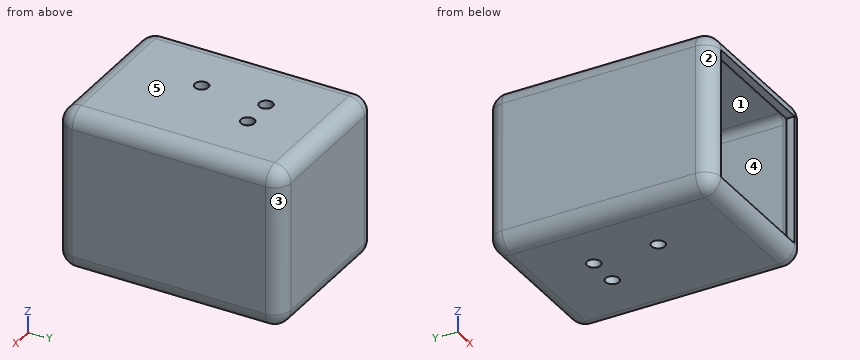
from build123d import *

# Parameters (mm, degrees)
F1_DEPTH = 35
F2_R     = 5
F3_T     = -2.5
F5_D     = 4.2


# Not quite as in the source:
# - a shell that OpenCascade refuses in one call is made with other operations: the cavity is built on its own and cut out


with BuildPart() as f1:
    # F0 (on Front) → F1 (new body, symmetric)
    with BuildSketch(Plane.XZ):
        with BuildLine():
            Line((20, 25), (-20, 25))
            ThreePointArc((-20, 25), (-23.5355339059, 23.5355339059), (-25, 20))
            Line((-25, 20), (-25, -20))
            ThreePointArc((-25, -20), (-23.5355339059, -23.5355339059), (-20, -25))
            Line((-20, -25), (20, -25))
            ThreePointArc((20, -25), (23.5355339059, -23.5355339059), (25, -20))
            Line((25, -20), (25, 20))
            ThreePointArc((25, 20), (23.5355339059, 23.5355339059), (20, 25))
        make_face()
    extrude(amount=F1_DEPTH, both=True)

    # F2
    f2_edges = [f1.edges().sort_by_distance(p)[0] for p in [
        (0, 35, 25),
        (-23.535534, 35, 23.535534),
        (-25, 35, 0),
        (-23.535534, 35, -23.535534),
        (0, 35, -25),
        (23.535534, 35, -23.535534),
        (25, 35, 0),
        (23.535534, 35, 23.535534),
        (0, -35, 25),
        (-23.535534, -35, 23.535534),
        (-25, -35, 0),
        (-23.535534, -35, -23.535534),
        (0, -35, -25),
        (23.535534, -35, -23.535534),
        (25, -35, 0),
        (23.535534, -35, 23.535534),
    ]]
    fillet(f2_edges, radius=F2_R)

    # F3: a shell. OpenCascade refuses it in one call, so the cavity is built on its own and cut out:
    # the body offset inwards by the wall thickness, plus a prism from it out through each open face.
    f3_core = offset(f1.part, amount=F3_T, mode=Mode.PRIVATE)
    f3_exits = [f3_core.faces().sort_by_distance(p)[0] for p in [
        (0, -32.5, 0),
    ]]
    add(f3_core, mode=Mode.SUBTRACT)
    extrude(f3_exits, amount=-F3_T, mode=Mode.SUBTRACT)

    # F5 (through all)
    with Locations(Plane(origin=(0, 0, -25), x_dir=(1, 0, 0), z_dir=(0, 0, -1))):
        with Locations((5, -13), (-5, 7), (-5, -13)):
            Hole(F5_D / 2)


solid = f1.part
For this review, take the finished solid that the model builds, in its own axes (mm). Face numbers are marked on the shaded views. A direction names the side the tool comes from. Round coordinates to 2 decimals unless told otherwise and drop trailing zeros. Write each loop counter-clockwise with the first axis right and the second up, starting at its lowest first coordinate (ties: lowest second). Pieces come first, ordered by that corner, then holes. Notation, with made-up numbers: (-33.75, 24) -> (-18.75, 24) arc R19 ccw to (-18.75, 47) -> close; hole circle Ø11 at (87, 49). An arc over 180 degrees is marked (long way). Put each result on its own line as item: value.
Q1. Clearance check with flat-ended pins moving along their axes: pin 1 Ø2.5 at (x, y) = (-5, -7) entering from +Z; pin 2 Ø0.8 at (x, y) = (-7.5, -33.5) entering from -Z; pin 3 Ø3 at (y, z) = (-34.5, 6) entering from -X; pin 4 Ø3 at (x, y) = (-3, -34) entering from +Z. State where each tip first meets the part, or that it passes through.
Determined:
pin 1: passes through
pin 2: stops at z = -23.92
pin 3: stops at x = -24
pin 4: stops at z = 24.33
Q2. Consider section B-B on x = 5. State the section outline as (y, z) points.
Determined:
outline: (-35, -20) arc R5 ccw to (-30, -25) -> (10.9, -25) -> (10.9, -22.5) -> (-30, -22.5) arc R2.5 cw to (-32.5, -20) -> close; (-35, 20) -> (-32.5, 20) arc R2.5 cw to (-30, 22.5) -> (10.9, 22.5) -> (10.9, 25) -> (-30, 25) arc R5 ccw to start; (15.1, -25) -> (30, -25) arc R5 ccw to (35, -20) -> (35, 20) arc R5 ccw to (30, 25) -> (15.1, 25) -> (15.1, 22.5) -> (30, 22.5) arc R2.5 cw to (32.5, 20) -> (32.5, -20) arc R2.5 cw to (30, -22.5) -> (15.1, -22.5) -> close
Q3. The part is to be moulded in two halves that separate along Z. For the marked faces 3, 4 and 5, say which applies: released by +Z, released by -Z, zero draft, split by the parting line, or undercut.
Determined:
face 3: zero draft
face 4: undercut
face 5: released by +Z
Q4. To check wall thickness, follow L1, parallel to Z at x = 17, y = 10; L2, parallel to X at y = 13, z = -23.95; L3, parallel to Y at x = -5, z = 24. State the ranges of each line that lie inside material, in increasing order. Write a range as [from, to].
Determined:
L1: z = [-25, -22.5], [22.5, 25]
L2: x = [-23.07, -7.1], [-2.9, 2.9], [7.1, 23.07]
L3: y = [-33, -9.1], [-4.9, 10.9], [15.1, 33]
Q5. Consider section A-A on y = -7. State the section outline as (x, z) points, and give its area (3 significant figures).
Determined:
outline: (-25, -20) arc R5 ccw to (-20, -25) -> (-7.1, -25) -> (-7.1, -22.5) -> (-20, -22.5) arc R2.5 cw to (-22.5, -20) -> (-22.5, 20) arc R2.5 cw to (-20, 22.5) -> (-7.1, 22.5) -> (-7.1, 25) -> (-20, 25) arc R5 ccw to (-25, 20) -> close; (-2.9, -25) -> (20, -25) arc R5 ccw to (25, -20) -> (25, 20) arc R5 ccw to (20, 25) -> (-2.9, 25) -> (-2.9, 22.5) -> (20, 22.5) arc R2.5 cw to (22.5, 20) -> (22.5, -20) arc R2.5 cw to (20, -22.5) -> (-2.9, -22.5) -> close
area: 438 mm^2
Q6. Consider section C-C on y = 13. Give the number of separate pieces and of enclosed holes in the cut face, and give its area (3 significant figures).
Determined:
separate pieces: 4
enclosed holes: 0
area: 417 mm^2
Q7. Machinability: for the marked faces 1 and 2, which of the approach directions +Z, -Z, +X, -X, +Y, -Y give a long, thin tool a straight path to every point of the face, cutting with its end or side? Answer none if there is none.
Determined:
face 1: none
face 2: +Z, -Z, -X, -Y
